from build123d import *

# Parameters (mm, degrees)
SKETCH_R        = 2.25
SKETCH_R_2      = 11.25
SKETCH_R_3      = 1.75
PAD_DEPTH       = 23
SKETCH001_R     = 4
POCKET_DEPTH    = 19
SKETCH002_R     = 2.25
POCKET001_DEPTH = 10
SKETCH003_R     = 4.05
POCKET002_DEPTH = 12
SKETCH004_R     = 3.75
POCKET003_DEPTH = 10


with BuildPart() as pocket002:
    # Sketch → Pad (new body)
    with BuildSketch(Plane.XY):
        Polygon((0, 0), (105, 0), (105, 62), (20, 62), (20, 42), (0, 42), align=None)
        with Locations((35, 10)):
            Circle(SKETCH_R, mode=Mode.SUBTRACT)
        with Locations((30, 35)):
            Circle(SKETCH_R, mode=Mode.SUBTRACT)
        with Locations((84, 21)):
            Circle(SKETCH_R_2, mode=Mode.SUBTRACT)
        with Locations((68.5, 36.5)):
            Circle(SKETCH_R_3, mode=Mode.SUBTRACT)
        with Locations((99.5, 36.5)):
            Circle(SKETCH_R_3, mode=Mode.SUBTRACT)
        with Locations((68.5, 5.5)):
            Circle(SKETCH_R_3, mode=Mode.SUBTRACT)
        with Locations((99.5, 5.5)):
            Circle(SKETCH_R_3, mode=Mode.SUBTRACT)
        with Locations((10, 30)):
            Circle(SKETCH_R, mode=Mode.SUBTRACT)
        with Locations((10, 15)):
            Circle(SKETCH_R, mode=Mode.SUBTRACT)
        with Locations((39, 52)):
            Circle(SKETCH_R, mode=Mode.SUBTRACT)
        with Locations((94, 52)):
            Circle(SKETCH_R, mode=Mode.SUBTRACT)
    extrude(amount=PAD_DEPTH)

    # Sketch001 → Pocket (cut)
    with BuildSketch(Plane.XY.offset(23)):
        with BuildLine():
            ThreePointArc((38.485281, 42), (36.015595, 44.209377), (32.999996, 45.583006))
            Line((32.999996, 67), (32.999996, 45.583006))
            Line((20, 67), (32.999996, 67))
            Line((20, -1), (20, 67))
            Line((20, -1), (48.252269, -1))
            Line((48.252269, 11), (48.252269, -1))
            Line((48.252269, 11), (70.252269, 11))
            ThreePointArc((70.252269, 11), (71.759618, 9.202833), (73.499996, 7.630258))
            Line((73.499996, 7.630258), (73.499996, -1))
            Line((73.499996, -1), (93.499996, -1))
            Line((93.499996, -1), (93.499996, 6.902128))
            ThreePointArc((93.499996, 6.902128), (95.574295, 8.548671), (97.367695, 10.497399))
            Line((105.499996, 10.497399), (97.367695, 10.497399))
            Line((105.499996, 30.497399), (105.499996, 10.497399))
            Line((98.099621, 30.497399), (105.499996, 30.497399))
            ThreePointArc((98.099621, 30.497399), (91.98574, 36.007594), (83.999996, 38))
            Line((83.999996, 38), (83.999996, 67))
            Line((83.999996, 67), (43.999996, 67))
            Line((43.999996, 67), (43.999996, 42))
            Line((38.485281, 42), (43.999996, 42))
        make_face()
        with Locations((68.5, 36.5)):
            Circle(SKETCH001_R, mode=Mode.SUBTRACT)
    extrude(amount=-POCKET_DEPTH, mode=Mode.SUBTRACT)

    # Sketch002 → Pocket001 (cut)
    with BuildSketch(Plane.XY.offset(23)):
        with Locations((55, 5)):
            Circle(SKETCH002_R)
    extrude(amount=-POCKET001_DEPTH, mode=Mode.SUBTRACT)

    # Sketch003 → Pocket002 (cut)
    with BuildSketch(Plane.XZ):
        with Locations((13, 16)):
            Circle(SKETCH003_R)
    extrude(amount=-POCKET002_DEPTH, mode=Mode.SUBTRACT)


with BuildPart() as pocket003:
    # Part__Mirroring: instance of Pocket002
    add(pocket002.part.mirror(Plane(origin=(0, 0, 0), x_dir=(0, -1, 0), z_dir=(1, 0, 0))))

    # Sketch004 → Pocket003 (cut)
    with BuildSketch(Plane(origin=(0, 0, 0), x_dir=(1, 0, 0), z_dir=(0, 0, -1))):
        with Locations((-10, -15)):
            Circle(SKETCH004_R)
        with Locations((-10, -30)):
            Circle(SKETCH004_R)
        with Locations((-94, -52)):
            Circle(SKETCH004_R)
        with Locations((-39, -52)):
            Circle(SKETCH004_R)
    extrude(amount=-POCKET003_DEPTH, mode=Mode.SUBTRACT)


solid = pocket003.part
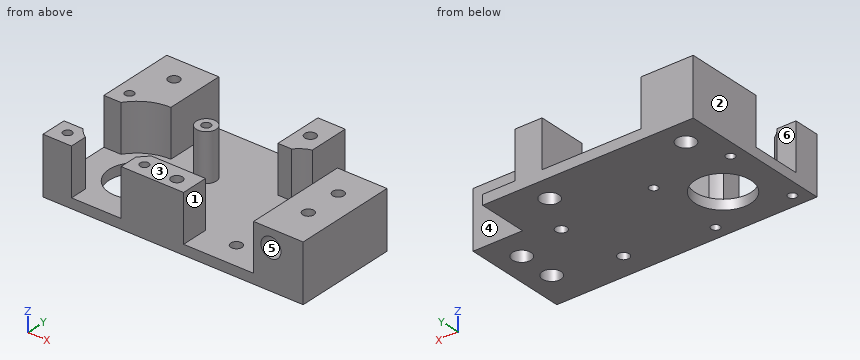
Read the model definition and answer for the solid it produces. Units are mm, in the model's axes. Face numbers are marked on the shaded views. A direction names the side the tool comes from. Coordinates: 2 decimals unless noted, no trailing zeros. Order: outer loops, then holes, each group sorted by start corner. A loop starts at its lowest first (then second) coordinate and runs counter-clockwise, first axis right, second up. Notation, with made-up numbers: M -31.5,44.25 L -9.5,44.25 A17 cw -9.5,76.25 Z; hole C -32.75,46.25 d4. An arc over 180 degrees is marked long. Put each result on its own line as item: value. Start each with the question number.
Item 1: Section B-B, the plane z = 2.5 is taken. Count the separate pieces of the cut face and the enclosed holes in it, plus the area to 3 significant figures.
Item 2: Given pin 1 Ø5 at (x, y) = (-92, 9) entering from +Z; pin 2 Ø1 at (y, z) = (20.5, 16) entering from -X; pin 3 Ø1.7 at (x, z) = (-41.5, 12) entering from -Y, each flat-ended and moving along its own axis, determine where each tip first touches the part or whether it passes through.
Item 3: Section A-A, the plane x = -68.5 is taken. Determine the outline of the cut face in (y, z), plus the area to 3 significant figures.
Item 4: Section D-D, the plane x = -99.5 is taken. Determine the outline of the cut face in (y, z), plus the area to 3 significant figures.
Item 5: The mould has two halves that part along X. Classify the marked faces 1, 2 and 3: +X half, -X half, draft (parallel to the pull), parting line (faces both ways), or undercut.
Item 6: For the marked faces 4, 5 and 6, determine the directions among +Z, -Z, +X, -X, +Y, -Y from which every point of the face is accessible in a straight line to the end or side of a thin tool.
Item 7: Consider probe 1 along Y at (x, z) = (-68.5, 6.5); probe 2 along Y at (x, z) = (-99.5, 16.75); probe 3 along X at (y, z) = (15, 6.25). Determine where each line is inside the solid, lowest interval first. Write a range as [from, to].
Computed:
1. separate pieces: 1
1. enclosed holes: 11
1. area: 5,470 mm2
2. pin 1: stops at z = 4
2. pin 2: stops at x = -20
2. pin 3: stops at y = 42
3. outline: M 0,0 L 3.75,0 L 3.75,23 L 0,23 Z; M 7.25,0 L 34.75,0 L 34.75,23 L 32.5,23 L 32.5,4 L 11,4 L 11,23 L 7.25,23 Z; M 38.25,0 L 62,0 L 62,4 L 40.5,4 L 40.5,23 L 38.25,23 Z
3. area: 448 mm2
4. outline: M 0,0 L 3.75,0 L 3.75,23 L 0,23 Z; M 7.25,0 L 34.75,0 L 34.75,23 L 30.5,23 L 30.5,4 L 10.5,4 L 10.5,23 L 7.25,23 Z; M 38.25,0 L 62,0 L 62,23 L 38.25,23 Z
4. area: 885 mm2
5. face 1: undercut
5. face 2: -X half
5. face 3: draft
6. face 4: +Z, -Z, +X, +Y
6. face 5: -Y
6. face 6: +Z, -X
7. probe 1: y = [0, 3.75], [7.25, 11], [32.5, 34.75], [38.25, 40.5]
7. probe 2: y = [0, 3.75], [7.25, 10.5], [30.5, 34.75], [38.25, 62]
7. probe 3: x = [-20, -13.75], [-6.25, 0]
